For this review, take the finished solid that the model builds, in its own axes (mm). A direction names the side the tool comes from. Give positions to 0.01 mm unless a question says otherwise; leave off trailing zeros. Loops run counter-clockwise (first coordinate to the right, second up) from the corner with the lowest first, then second, coordinate; pieces in that order, holes last.
```python
from build123d import *

# Parameters (mm, degrees)
SKETCH_W        = 664
SKETCH_H        = 380
PAD_DEPTH       = 25
SKETCH001_W     = 644
SKETCH001_H     = 360
POCKET_DEPTH    = 10
SKETCH002_W     = 65
SKETCH002_H     = 10
PAD001_DEPTH    = 73
SKETCH003_R     = 8
POCKET001_DEPTH = 10
SKETCH004_W     = 65
SKETCH004_H     = 15
PAD002_DEPTH    = 83
SKETCH005_R     = 8
POCKET002_DEPTH = 100
SKETCH006_W     = 40
SKETCH006_H     = 60
PAD003_DEPTH    = 15


with BuildPart() as part:
    # Sketch → Pad (new body)
    with BuildSketch(Plane.XY):
        Rectangle(SKETCH_W, SKETCH_H)
    extrude(amount=PAD_DEPTH)

    # Sketch001 (on Face6 of Pad) → Pocket (cut)
    with BuildSketch(Plane.XY.offset(25)):
        Rectangle(SKETCH001_W, SKETCH001_H)
    extrude(amount=-POCKET_DEPTH, mode=Mode.SUBTRACT)

    # Sketch002 (on Face5 of Pocket) → Pad001 (join)
    with BuildSketch(Plane.XY.offset(25)):
        with Locations((-249, -185)):
            Rectangle(SKETCH002_W, SKETCH002_H)
        with Locations((-83, -185)):
            Rectangle(SKETCH002_W, SKETCH002_H)
        with Locations((83, -185)):
            Rectangle(SKETCH002_W, SKETCH002_H)
        with Locations((249, -185)):
            Rectangle(SKETCH002_W, SKETCH002_H)
    extrude(amount=PAD001_DEPTH)

    # Sketch003 (on Face25 of Pad001) → Pocket001 (cut)
    with BuildSketch(Plane.XZ.offset(190)):
        with Locations((249, 60)):
            Circle(SKETCH003_R)
        with Locations((83, 60)):
            Circle(SKETCH003_R)
        with Locations((-83, 60)):
            Circle(SKETCH003_R)
        with Locations((-249, 60)):
            Circle(SKETCH003_R)
    extrude(amount=-POCKET001_DEPTH, mode=Mode.SUBTRACT)

    # Sketch004 (on Face27 of Pocket001) → Pad002 (join)
    with BuildSketch(Plane.XY.offset(15)):
        with Locations((249, -97.5)):
            Rectangle(SKETCH004_W, SKETCH004_H)
        with Locations((83, -97.5)):
            Rectangle(SKETCH004_W, SKETCH004_H)
        with Locations((-249, -97.5)):
            Rectangle(SKETCH004_W, SKETCH004_H)
        with Locations((-83, -97.5)):
            Rectangle(SKETCH004_W, SKETCH004_H)
    extrude(amount=PAD002_DEPTH)

    # Sketch005 → Pocket002 (cut)
    with BuildSketch(Plane.XZ.offset(190)):
        with Locations((-249, 60)):
            Circle(SKETCH005_R)
        with Locations((-83, 60)):
            Circle(SKETCH005_R)
        with Locations((83, 60)):
            Circle(SKETCH005_R)
        with Locations((249, 60)):
            Circle(SKETCH005_R)
    extrude(amount=-POCKET002_DEPTH, mode=Mode.SUBTRACT)

    # Sketch006 (on Face27 of Pocket002) → Pad003 (join)
    with BuildSketch(Plane.XY.offset(15)):
        with Locations((-249, -30)):
            Rectangle(SKETCH006_W, SKETCH006_H)
        with Locations((-83, -30)):
            Rectangle(SKETCH006_W, SKETCH006_H)
        with Locations((83, -30)):
            Rectangle(SKETCH006_W, SKETCH006_H)
        with Locations((249, -30)):
            Rectangle(SKETCH006_W, SKETCH006_H)
    extrude(amount=PAD003_DEPTH)


solid = part.part
```
Q1. Mouldability with a two-part tool opening along Z and no side actions: class faces 1 (the flat face through (-5, 190, 12)), 2 (the flat face through (-5, 3, 0)), 3 (the cylindrical face through (81.959, -97.605, 67.932)), 4 (the flat face through (83, -30, 30)) as +Z half, -Z half, draft (parallel to the pull), parting line (faces both ways), or undercut.
Answers:
face 1: draft
face 2: -Z half
face 3: undercut
face 4: +Z half
Q2. For pin 1 Ø3 at (y, z) = (-185.5, 65) entering from +X; pin 2 Ø6 at (x, y) = (-83, -9.5) entering from +Z; pin 3 Ø1 at (x, z) = (-88, 82) entering from +Y, all flat-tipped, find the tip position at first contact; note any pin that passes through.
Answers:
pin 1: stops at x = 281.5
pin 2: stops at z = 30
pin 3: stops at y = -90
Q3. Consider section C-C on y = 44.5. Give the boundary of the cut face in (x, z), plus the area to 3 significant figures.
Answers:
outline: (-332, 0) - (332, 0) - (332, 25) - (322, 25) - (322, 15) - (-322, 15) - (-322, 25) - (-332, 25) - close
area: 10,200 mm2
Q4. For probe 1 along Y at (x, z) = (85.5, 16); probe 2 along Z at (x, y) = (249, -184.25); probe 3 along X at (y, z) = (-137, 17.5), list the stretches that pass through material, from the lowest coordinate up.
Answers:
probe 1: y = -190 to -180, -105 to -90, -60 to 0, 180 to 190
probe 2: z = 0 to 52, 68 to 98
probe 3: x = -332 to -322, 322 to 332
Q5. Consider section A-A on z = 84. Count the separate pieces of the cut face and the enclosed holes in it, plus the area to 3 significant figures.
Answers:
separate pieces: 8
enclosed holes: 0
area: 6,500 mm2
Q6. Machinability: for faces 5 (the flat face through (229, -30, 22)), 6 (the flat face through (-249, -30, 30)), 7 (the cylindrical face through (-84.041, -185.07, 67.932)), which of the approach directions +Z, -Z, +X, -X, +Y, -Y give a long, thin tool a straight path to every point of the face, cutting with its end or side? Answer none if there is none.
Answers:
face 5: +Z
face 6: +Z, +X, -X, +Y
face 7: +Y, -Y
Q7. Consider section B-B on x = -83. Give the boundary of the cut face in (y, z), plus the area to 4 significant figures.
Answers:
outline: (-190, 0) - (190, 0) - (190, 25) - (180, 25) - (180, 15) - (0, 15) - (0, 30) - (-60, 30) - (-60, 15) - (-90, 15) - (-90, 52) - (-105, 52) - (-105, 15) - (-180, 15) - (-180, 52) - (-190, 52) - close; (-190, 68) - (-180, 68) - (-180, 98) - (-190, 98) - close; (-105, 68) - (-90, 68) - (-90, 98) - (-105, 98) - close
area: 8,375 mm2
